Part model, mm, in its own coordinate system. Face numbers are marked on the shaded views. A direction names the side the tool comes from. Round coordinates to 2 decimals unless told otherwise and drop trailing zeros. Loops run counter-clockwise (first coordinate to the right, second up) from the corner with the lowest first, then second, coordinate; pieces in that order, holes last. Notation, with made-up numbers: (20, 35) -> (45, 35) arc R19 cw to (45, 53) -> close; hole circle Ø4 at (20.25, 57). An arc over 180 degrees is marked (long way). Use a Markdown table: item, result. Add a question column.
Item 1: Which spindle directions (+Z, -Z, +X, -X, +Y, -Y) get a long thin tool onto all of the face, cutting with end or side? Do the marked faces 1, 2 and 3. Say none if no direction does.
Item 2: Probe line 1 (Y direction, x = 0, z = -4.25); line 2 (Y direction, x = -1, z = -7.75); line 3 (Y direction, x = -31, z = 11.5). List the from-to ranges inside material, lowest first. Write a range as [from, to].
Item 3: Cut at D-D, the plane x = 20.5. List the corners of the cut face in (y, z).
Item 4: Cut at B-B, the plane z = 12.75. List the corners of the cut face in (x, y), plus the area to 3 significant figures.
Item 5: Cut at C-C, the plane y = 113. List the corners of the cut face in (x, z), plus the area to 3 significant figures.
Item 6: Cut at A-A, the plane x = 0. List the corners of the cut face in (y, z), plus the area to 3 significant figures.
Item 7: Two-plate mould, pull along Y, no slides. Class the marked faces 4, 5 and 6: pulls with the +Y half, pulls with the -Y half, needs draft (parallel to the pull), parting line crosses it, or undercut.
Item 8: Flat gauge pins, fed straight in: pin 1 (1.5 mm diameter, centred on x = -2, y = 45, fed in from -Z); pin 2 (13 mm diameter, centred on x = -24.5, z = 1.5, fed in from +Y); pin 3 (9.5 mm diameter, centred on x = 28, z = -1, fed in from +Y); pin 4 (12 mm diameter, centred on x = 19, z = -4, fed in from -Y). Where does each tip first touch, or does it go through?
```python
from build123d import *

# Parameters (mm, degrees)
BOSS_EXTRUDE1_DEPTH = 15
BOSS_EXTRUDE2_REACH = 44.119
SKETCH4_R           = 3.25
CUT_EXTRUDE1_DEPTH  = 43.118879377
BOSS_EXTRUDE3_DEPTH = 7.5
CUT_EXTRUDE2_DEPTH  = 2
SKETCH9_R           = 12.5
SKETCH9_R_2         = 9
BOSS_EXTRUDE4_DEPTH = 10


with BuildPart() as part:
    # Sketch1 → Boss-Extrude1 (new, symmetric)
    with BuildSketch(Plane.XY):
        with BuildLine():
            Line((-22.5, 0), (-35, 0))
            Line((-35, 0), (-35, 3))
            Line((-35, 3), (-25.322914524, 3))
            ThreePointArc((-25.322914524, 3), (0, 25.5), (25.322914524, 3))
            Line((25.322914524, 3), (35, 3))
            Line((35, 3), (35, 0))
            Line((35, 0), (22.5, 0))
            ThreePointArc((22.5, 0), (0, 22.5), (-22.5, 0))
        make_face()
    extrude(amount=BOSS_EXTRUDE1_DEPTH, both=True)

    # Sketch3 → Boss-Extrude2 (add, up to next)
    with BuildSketch(Plane(origin=(0, 18, 0), x_dir=(1, 0, 0), z_dir=(0, 1, 0)), mode=Mode.PRIVATE) as boss_extrude2_sk1:
        with BuildLine():
            Line((-18.06, 6), (-18.06, -6))
            Line((-18.06, -6), (-29, -6))
            ThreePointArc((-29, -6), (-35, 0), (-29, 6))
            Line((-29, 6), (-18.06, 6))
        make_face()
    boss_extrude2_tool1 = extrude(boss_extrude2_sk1.sketch, amount=-BOSS_EXTRUDE2_REACH, mode=Mode.PRIVATE) - part.part
    boss_extrude2 = boss_extrude2_tool1.solids().sort_by_distance((-25.943483, 18, 0))[0]
    add(boss_extrude2)

    # Sketch4 → Cut-Extrude1 (cut, through all)
    with BuildSketch(Plane(origin=(0, 18, 0), x_dir=(1, 0, 0), z_dir=(0, 1, 0))):
        with Locations(Location((-29, 0, 0), (0, 0, 180))):
            Circle(SKETCH4_R)
    cut_extrude1 = extrude(amount=-CUT_EXTRUDE1_DEPTH, mode=Mode.SUBTRACT)

    # Mirror1: Boss-Extrude2, Cut-Extrude1 across plane
    add(boss_extrude2.mirror(Plane(origin=(0, 0, 0), x_dir=(0, 0, 1), z_dir=(1, 0, 0))))
    add(cut_extrude1.mirror(Plane(origin=(0, 0, 0), x_dir=(0, 0, 1), z_dir=(1, 0, 0))), mode=Mode.SUBTRACT)

    # Sketch6 → Boss-Extrude3 (add, symmetric)
    with BuildSketch(Plane.XY):
        with BuildLine():
            Line((15.957377604, 19.89), (8.003783203, 110.8))
            ThreePointArc((8.003783203, 110.8), (0, 107.901533963), (-8.003783203, 110.8))
            Line((-8.003783203, 110.8), (-15.957377604, 19.89))
            ThreePointArc((-15.957377604, 19.89), (0, 25.5), (15.957377604, 19.89))
        make_face()
    extrude(amount=BOSS_EXTRUDE3_DEPTH, both=True)

    # Sketch7 → Cut-Extrude2 (cut)
    with BuildSketch(Plane.XY.offset(7.5)):
        with BuildLine():
            Line((-5.422676431, 105.881045668), (-12.442830342, 25.640319286))
            ThreePointArc((-12.442830342, 25.640319286), (0, 28.5), (12.442830342, 25.640319286))
            Line((12.442830342, 25.640319286), (5.422676431, 105.881045668))
            ThreePointArc((5.422676431, 105.881045668), (0, 104.901533963), (-5.422676431, 105.881045668))
        make_face()
    cut_extrude2 = extrude(amount=-CUT_EXTRUDE2_DEPTH, mode=Mode.SUBTRACT)

    # Mirror2: Cut-Extrude2 across plane
    add(cut_extrude2.mirror(Plane.XY), mode=Mode.SUBTRACT)

    # Sketch9 → Boss-Extrude4 (add, symmetric)
    with BuildSketch(Plane.XY):
        with Locations((0, 120.401533963)):
            Circle(SKETCH9_R)
        with Locations((0, 120.401533963)):
            Circle(SKETCH9_R_2, mode=Mode.SUBTRACT)
    extrude(amount=BOSS_EXTRUDE4_DEPTH, both=True)


solid = part.part
```
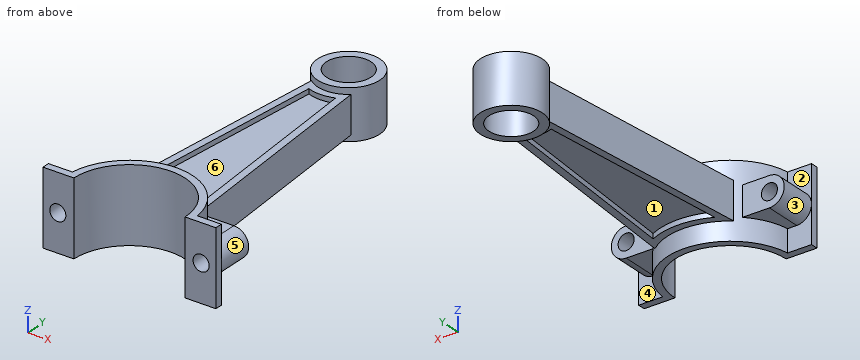
A:
| question | item | result |
|---|---|---|
| 1 | face 1 | -Z |
| 1 | face 2 | +Z, -X, +Y |
| 1 | face 3 | -X, +Y |
| 2 | line 1 | y = [22.5, 111.4], [129.4, 132.9] |
| 2 | line 2 | y = [22.48, 25.48], [107.94, 111.46], [129.35, 132.86] |
| 2 | line 3 | y = [0, 3] |
| 3 | outline | (9.27, -15) -> (15.17, -15) -> (15.17, -6) -> (18, -6) -> (18, 6) -> (15.17, 6) -> (15.17, 15) -> (9.27, 15) -> close |
| 4 | outline | (-35, 0) -> (-22.5, 0) arc R22.5 cw to (22.5, 0) -> (35, 0) -> (35, 3) -> (25.32, 3) arc R25.5 ccw to (-25.32, 3) -> (-35, 3) -> close |
| 4 | area | 284 mm^2 |
| 5 | outline | (-10.07, -10) -> (-5.12, -10) -> (-5.12, 10) -> (-10.07, 10) -> close; (5.12, -10) -> (10.07, -10) -> (10.07, 10) -> (5.12, 10) -> close |
| 5 | area | 198 mm^2 |
| 6 | outline | (22.5, -15) -> (25.5, -15) -> (25.5, -7.5) -> (28.5, -7.5) -> (28.5, -5.5) -> (104.9, -5.5) -> (104.9, -7.5) -> (107.9, -7.5) -> (107.9, -10) -> (111.4, -10) -> (111.4, 10) -> (107.9, 10) -> (107.9, 7.5) -> (104.9, 7.5) -> (104.9, 5.5) -> (28.5, 5.5) -> (28.5, 7.5) -> (25.5, 7.5) -> (25.5, 15) -> (22.5, 15) -> close; (129.4, -10) -> (132.9, -10) -> (132.9, 10) -> (129.4, 10) -> close |
| 6 | area | 1,160 mm^2 |
| 7 | face 4 | pulls with the +Y half |
| 7 | face 5 | needs draft |
| 7 | face 6 | undercut |
| 8 | pin 1 | stops at z = -5.5 |
| 8 | pin 2 | stops at y = 18.06 |
| 8 | pin 3 | stops at y = 18 |
| 8 | pin 4 | stops at y = 0 |
